from build123d import *

# Parameters (mm, degrees)
SZKIC1_R                    = 5
DODANIE_WYCI_GNI_CIE1_DEPTH = 25
DODANIE_WYCI_GNI_CIE2_DEPTH = 6
ZAOKR_GLENIE1_R             = 0.5


with BuildPart() as part:
    # Szkic1 → Dodanie-wyciągnięcie1 (new body)
    with BuildSketch(Plane(origin=(0, 0, 0), x_dir=(1, 0, 0), z_dir=(0, 1, 0))):
        Circle(SZKIC1_R)
    extrude(amount=DODANIE_WYCI_GNI_CIE1_DEPTH)

    # Szkic2 → Dodanie-wyciągnięcie2 (add)
    with BuildSketch(Plane(origin=(0, 0, 0), x_dir=(-1, 0, 0), z_dir=(0, -1, 0))):
        Polygon((-0.721110691, -9.78842851), (8.116472407, -5.518714433), (8.837583099, 4.269714077), (0.721110691, 9.78842851), (-8.116472407, 5.518714433), (-8.837583099, -4.269714077), align=None)
    extrude(amount=DODANIE_WYCI_GNI_CIE2_DEPTH)

    # Zaokrąglenie1
    zaokr_glenie1_edges = [part.edges().sort_by_distance(p)[0] for p in [
        (-5, 0, 0),
    ]]
    fillet(zaokr_glenie1_edges, radius=ZAOKR_GLENIE1_R)


solid = part.part
Part model, mm, in its own coordinate system. A direction names the side the tool comes from. Round coordinates to 2 decimals unless told otherwise and drop trailing zeros. Write each loop counter-clockwise with the first axis right and the second up, starting at its lowest first coordinate (ties: lowest second). Pieces come first, ordered by that corner, then holes. Notation, with made-up numbers: M 14,-31 L 22,-31 A21 cw 22,-14 Z; hole C 48.25,-29 d4. An arc over 180 degrees is marked long. Return JSON: item names as keys, results as strings. Group by question number.
(1) Saw through at A-A on x = 0. Write the cut outline in (y, z).
(2) Which spindle directions (+Z, -Z, +X, -X, +Y, -Y) get a long thin tool onto all of the face, cutting with end or side? Do faces 1 (the face through (-1.08, 12.58, 4.88)), 2 (the face through (-3.6, -3, 7.7)). Say none if no direction does.
(3) Drill centre lines: probe 1 along Y at (x, z) = (-2, -5.75); probe 2 along X at (y, z) = (20, -0.25); probe 3 along X at (y, z) = (12.5, 1.5). Where is each one in solid material? Low to high.
(4) Saw through at D-D on y = 4. Write the cut outline in (x, z), then the cut area to 3 significant figures.
(5) Saw through at C-C on z = 0. Write the cut outline in (x, y), then the cut area to 3 significant figures.
(6) Pin check, flat tips, straight feed: pin 1 Ø10 at (x, y) = (-5, -0.5) entering from +Z; pin 2 Ø1.5 at (y, z) = (13.5, 4.5) entering from +X; pin 3 Ø6 at (y, z) = (9, 0.5) entering from +X. Stop position of each tip, or through.
(7) Saw through at B-B on y = -3. Write the cut outline in (x, z).
Returned:
{
 "1": {"outline": "M -6,-9.44 L 0,-9.44 L 0,-5.5 A0.5 cw 0.5,-5 L 25,-5 L 25,5 L 0.5,5 A0.5 cw 0,5.5 L 0,9.44 L -6,9.44 Z"},
 "2": {"face 1": "+Y", "face 2": "+Z, -X, +Y, -Y"},
 "3": {"probe 1": "-6 to 0", "probe 2": "-4.99 to 4.99", "probe 3": "-4.77 to 4.77"},
 "4": {"outline": "C 0,0 d10", "area": "78.5 mm²"},
 "5": {"outline": "M -8.52,-6 L 8.52,-6 L 8.52,0 L 5.5,0 A0.5 cw 5,0.5 L 5,25 L -5,25 L -5,0.5 A0.5 cw -5.5,0 L -8.52,0 Z", "area": "352 mm²"},
 "6": {"pin 1": "z = 9.44", "pin 2": "x = 3.31", "pin 3": "x = 5"},
 "7": {"outline": "M -8.84,-4.27 L -0.72,-9.79 L 8.12,-5.52 L 8.84,4.27 L 0.72,9.79 L -8.12,5.52 Z"}
}
